Check sheet for the modelled part. Datum: model origin and axes. Units: mm. A direction names the side the tool comes from. Give positions to 0.01 mm unless a question says otherwise; leave off trailing zeros. Loops run counter-clockwise (first coordinate to the right, second up) from the corner with the lowest first, then second, coordinate; pieces in that order, holes last. Notation, with made-up numbers: (72.5, -21.5) -> (130.5, -21.5) arc R22 ccw to (130.5, 8.5) -> close; hole circle Ø9 at (-19, -17.75). An arc over 180 degrees is marked (long way). Write each question's results on one line, items separated by ' | '. Start each with the question number.
Item 1: Cross-section at B-B on x = -4. Enter the section's corners in (y, z), then the cut area to 3 significant figures.
Item 2: Scan line: line 1 along Z through (x, y) = (-25, 0.4). Record every from-to range of solid material in increasing order.
Item 3: Access from +Z, -Z, +X, -X, +Y, -Y to the whole of each face (thin tool, end or side, straight path). Record for faces 1 (the face through (-3, 3, -144.78)), 2 (the face through (-24.16, 3, -147)), 3 (the face through (-24.16, 3, 3)), 4 (the face through (-6.38, 3, 3)).
Item 4: Gauge pin test, flat ends, axial feed: pin 1 Ø1.5 at (y, z) = (1.5, -147.5) entering from -X; pin 2 Ø1.5 at (x, y) = (-28.5, 3) entering from -Z; pin 3 Ø1.5 at (x, y) = (-2, 3.5) entering from +Z. Record the tip position at first contact, or that the pin passes through.
Item 5: Cross-section at A-A on y = 1. Enter the section's corners in (x, z).
from build123d import *

# Parameters (mm, degrees)
SKETCH1_W           = 30.54
SKETCH1_H           = 144.78
BOSS_EXTRUDE1_DEPTH = 5.08
SKETCH2_W           = 17.78
SKETCH2_H           = 5.08
BOSS_EXTRUDE2_DEPTH = 5.08
SKETCH3_W           = 17.78
SKETCH3_H           = 5.08
BOSS_EXTRUDE3_DEPTH = 5.08


with BuildPart() as part:
    # Sketch1 → Boss-Extrude1 (new body)
    with BuildSketch(Plane(origin=(0, 0, 0), x_dir=(1, 0, 0), z_dir=(0, 1, 0))):
        with Locations((-15.27, 72.39)):
            Rectangle(SKETCH1_W, SKETCH1_H)
    extrude(amount=BOSS_EXTRUDE1_DEPTH)

    # Sketch2 → Boss-Extrude2 (add)
    with BuildSketch(Plane.XY):
        with Locations((-15.27, 2.54)):
            Rectangle(SKETCH2_W, SKETCH2_H)
    extrude(amount=BOSS_EXTRUDE2_DEPTH)

    # Sketch3 → Boss-Extrude3 (add)
    with BuildSketch(Plane(origin=(0, 0, -144.78), x_dir=(-1, 0, 0), z_dir=(0, 0, -1))):
        with Locations((15.27, 2.54)):
            Rectangle(SKETCH3_W, SKETCH3_H)
    extrude(amount=BOSS_EXTRUDE3_DEPTH)


solid = part.part
Answer sheet:
1) outline: (0, -144.78) -> (5.08, -144.78) -> (5.08, 0) -> (0, 0) -> close | area: 735 mm²
2) line 1: z = -144.78 to 0
3) face 1: -Z, +X, +Y, -Y | face 2: -Z, -X, +Y, -Y | face 3: +Z, -X, +Y, -Y | face 4: +Z, +X, +Y, -Y
4) pin 1: stops at x = -24.16 | pin 2: stops at z = -144.78 | pin 3: stops at z = 0
5) outline: (-30.54, -144.78) -> (-24.16, -144.78) -> (-24.16, -149.86) -> (-6.38, -149.86) -> (-6.38, -144.78) -> (0, -144.78) -> (0, 0) -> (-6.38, 0) -> (-6.38, 5.08) -> (-24.16, 5.08) -> (-24.16, 0) -> (-30.54, 0) -> close
